The model under review builds one solid part; all positions refer to its coordinate system, in mm. Coordinates: 2 decimals unless noted, no trailing zeros. Order: outer loops, then holes, each group sorted by start corner. A loop starts at its lowest first (then second) coordinate and runs counter-clockwise, first axis right, second up. Notation, with made-up numbers: (-29, -3) - (30, -3) arc R20 ccw to (30, 1) - close; hole circle Ø11 at (49.5, 29). An arc over 180 degrees is marked (long way). Answer in a Markdown table with one row per item.
Autodesk Inventor part; units mm, degrees
ref_plane "YZ Plane" through (0, 0, 0) normal (1, 0, 0) x (0, 1, 0)
ref_plane "XZ Plane" through (0, 0, 0) normal (0, 1, 0) x (-1, 0, 0)
ref_plane "XY Plane" through (0, 0, 0) normal (0, 0, 1) x (1, 0, 0)
sketch "Náčrt1" plane through (3.6, 12.9231, 50.0016) normal (0, 0, 1) x (1, 0, 0)
  line L0 (3.4, -51.2206) -> (3.4, 32.0765)
  line L1 (-10.6, 32.0765) -> (-10.6, -51.2206)
  line L2 (3.4, 32.0765) -> (-10.6, 32.0765)
  circle A0 centre (-3.5987, -48.8454) radius 2.0783
  line L3 (0, -50.927) -> (0, 0)
  line L4 (-3.6, -53.0054) -> (0, -50.927)
  line L5 (-7.2, -50.927) -> (-3.6, -53.0054)
  arc A1 (-10.6, -50.9238) -> (3.4, -50.787) centre (-3.5993, -50.9238) ccw
  line L6 (3.4, -25.4635) -> (3.4, -18.4635)
  line L7 (3.4, -18.4635) -> (23.4, -18.4635)
  line L8 (23.4, -18.4635) -> (23.4, -32.4635)
  line L9 (23.4, -32.4635) -> (3.4, -32.4635)
  line L10 (3.4, -25.4635) -> (3.4, -32.4635)
  line L11 (23.4, -25.4635) -> (23.4, -22.9635)
  line L12 (23.4, -22.9635) -> (26.9, -22.9635)
  line L13 (26.9, -22.9635) -> (26.9, -27.9635)
  line L14 (26.9, -27.9635) -> (23.4, -27.9635)
  line L15 (23.4, -25.4635) -> (23.4, -27.9635)
  line L16 (35.5188, -25.4635) -> (33.2094, -29.4635)
  line L17 (33.2094, -29.4635) -> (28.5906, -29.4635)
  line L18 (28.5906, -29.4635) -> (27.7246, -27.9635)
  line L19 (27.7246, -22.9635) -> (28.5906, -21.4635)
  line L20 (28.5906, -21.4635) -> (33.2094, -21.4635)
  line L21 (33.2094, -21.4635) -> (35.5188, -25.4635)
  line L22 (26.9, -22.9635) -> (27.7246, -22.9635)
  line L23 (26.9, -27.9635) -> (27.7246, -27.9635)
  line L24 (-10.6, -25.4635) -> (-10.6, -18.4635)
  line L25 (-10.6, -18.4635) -> (-30.6, -18.4635)
  line L26 (-30.6, -18.4635) -> (-30.6, -32.4635)
  line L27 (-30.6, -32.4635) -> (-10.6, -32.4635)
  line L28 (-10.6, -25.4635) -> (-10.6, -32.4635)
  line L29 (-30.6, -25.4635) -> (-30.6, -22.9635)
  line L30 (-30.6, -25.4635) -> (-30.6, -27.9635)
  line L31 (-27.1, -27.9635) -> (-30.6, -27.9635)
  line L32 (-30.6, -22.9635) -> (-27.1, -22.9635)
  line L33 (-27.1, -22.9635) -> (-27.1, -27.9635)
  line L34 (-27.1, -22.9635) -> (-26.2754, -22.9635)
  line L35 (-27.1, -27.9635) -> (-26.2754, -27.9635)
  line L36 (-25.4094, -29.4635) -> (-26.2754, -27.9635)
  line L37 (-26.2754, -22.9635) -> (-25.4094, -21.4635)
  line L38 (-20.7906, -29.4635) -> (-25.4094, -29.4635)
  line L39 (-25.4094, -21.4635) -> (-20.7906, -21.4635)
  line L40 (-18.4812, -25.4635) -> (-20.7906, -29.4635)
  line L41 (-20.7906, -21.4635) -> (-18.4812, -25.4635)
  line L42 (-3.6, 32.0765) -> (-3.6, 46.0765)
  arc A2 (-31.8843, 17.7922) -> (24.6843, 17.7922) centre (-3.6, 46.0765) ccw
  line L43 (-3.6, 46.0765) -> (-31.8843, 17.7922)
  line L44 (-3.6, 46.0765) -> (24.6843, 17.7922)
  line L45 (-3.6, 46.0765) -> (48.0562, 46.0765) construction
  line L46 (-25.5203, 24.1562) -> (-23.7525, 25.9239)
  line L47 (-25.5203, 24.1562) -> (-27.2881, 22.3884)
  line L48 (-24.8132, 19.9135) -> (-27.2881, 22.3884)
  line L49 (-23.7525, 25.9239) -> (-21.2777, 23.4491)
  line L50 (-21.2777, 23.4491) -> (-24.8132, 19.9135)
  line L51 (-21.2777, 23.4491) -> (-20.6946, 22.866)
  line L52 (-24.8132, 19.9135) -> (-24.2301, 19.3305)
  line L53 (-20.6946, 22.866) -> (-19.0216, 23.3143)
  line L54 (-24.6784, 17.6574) -> (-24.2301, 19.3305)
  line L55 (-19.0216, 23.3143) -> (-15.7556, 20.0483)
  line L56 (-16.951, 15.5869) -> (-21.4124, 14.3914)
  line L57 (-15.7556, 20.0483) -> (-16.951, 15.5869)
  line L58 (-21.4124, 14.3914) -> (-24.6784, 17.6574)
  line L59 (26.8896, 32.7254) -> (28.085, 28.264)
  line L60 (22.4282, 33.9209) -> (26.8896, 32.7254)
  line L61 (28.085, 28.264) -> (24.819, 24.998)
  line L62 (19.1622, 30.6549) -> (22.4282, 33.9209)
  line L63 (18.3203, 24.1562) -> (16.5525, 25.9239)
  line L64 (19.6105, 28.9819) -> (19.1622, 30.6549)
  line L65 (24.819, 24.998) -> (23.146, 25.4463)
  line L66 (19.0274, 28.3988) -> (19.6105, 28.9819)
  line L67 (19.0274, 28.3988) -> (22.563, 24.8633)
  line L68 (22.563, 24.8633) -> (23.146, 25.4463)
  line L69 (22.563, 24.8633) -> (20.0881, 22.3884)
  line L70 (18.3203, 24.1562) -> (20.0881, 22.3884)
  line L71 (16.5525, 25.9239) -> (19.0274, 28.3988)
  line L72 (24.6843, 17.7922) -> (18.3203, 24.1562)
  circle A3 centre (-3.6, 46.0765) radius 5
  line L73 (-7.2, -50.927) -> (-7.2, 32.0765)
  line L74 (0, -50.927) -> (0, 32.0765)
  line L75 (-7.2, 29.2565) -> (-3.6, 32.0765)
  line L76 (-3.6, 32.0765) -> (0, 29.2565)
  line L77 (-3.6, 29.2565) -> (-1.5215, 29.2565) construction
  circle A4 centre (-3.6, 27.178) radius 2.0785
  line L78 (-5.6785, 27.1779) -> (-5.677, -48.8455)
  line L79 (-1.5215, 27.1779) -> (-1.5203, -48.8454)
  point P0 (30.9, -25.4635)
  point P1 (26.9, -25.4635)
  point P2 (-27.1, -25.4635)
  point P3 (-23.1, -25.4635)
  point P4 (-23.0454, 21.6813)
  point P5 (-20.217, 18.8529)
  point P6 (23.4958, 25.7125)
  point P7 (23.6236, 29.4595)
  point P8 (20.7952, 26.631)
  point P9 (-10.6, 6.6937)
  point P10 (3.4, 6.6937)
  point P11 (16.5525, 25.9239)
  point P12 (-0.0645, 42.5409)
  point P13 (-7.1355, 42.5409)
  dimension "d4" = 7
  dimension "d5" = 20
  dimension "k" = 14
  dimension "d9" = 3.5
  dimension "d10" = 5
  dimension "d14" = 8
  dimension "d15" = 4
  dimension "d16" = 7
  dimension "d19" = 14
  dimension "d21" = 45
  dimension "d22" = 40
  dimension "d24" = 10
  dimension "d34" = 4.1567
  dimension "d35" = 2.0817
  dimension "d36" = 2.82
extrude "Vysunutí1" add sketch "Náčrt1" against normal blind 4 contours A1 L1 A2 L73 L5 L4 L3 L74 L0 | A2 L74 L2 L0 | L74 L3 L4 L5 L73 A2 L78 A0 L79 | A2 L79 A4 L78 L73 L75 L76 L74 | L1 L2 L73 A2 | L74 L76 L2 | L79 A0 L78 A2 | A2 L78 A4 L79 | L75 L73 L2 | A4 | A0
extrude "Vysunutí2" cut sketch "Náčrt1" against normal blind 2.5 contours L74 L3 L4 L5 L73 A2 L78 A0 L79 | A2 L79 A4 L78 L73 L75 L76 L74 | L79 A0 L78 A2 | A2 L78 A4 L79 | A4 | A0
extrude "Vysunutí3" add sketch "Náčrt1" against normal blind 4 contours L0 L7 L8 L9 | L27 L26 L31 L35 L36 L38 L40 L41 L39 L37 L34 L32 L25 L1 | L8 L12 L13 L14 | L13 L22 L19 L20 L21 L16 L17 L18 L23
extrude "Vysunutí4" add sketch "Náčrt1" against normal blind 4 contours L0 L2 L42 A3 L44 A2 | A2 L43 L48 L52 L54 L58 L56 L57 L55 L53 L51 L49 A3 L42 L2 L1 | L44 L71 L67 L69 | L67 L66 L64 L62 L60 L59 L61 L65 L68
sketch "Náčrt2" plane through (3.6, 12.9231, 50.0016) normal (0, 0, 1) x (1, 0, 0)
  line L0 (-7.2, 0) -> (-3.6, 2.0785)
  line L1 (-3.6, 2.0785) -> (0, 0)
  arc A0 (-1.525, -2.1008) -> (-5.675, -2.1796) centre (-3.6012, -2.0791) ccw
  line L2 (-5.675, -2.1796) -> (-5.675, -48.7542)
  line L3 (-1.525, -48.7062) -> (-1.525, -2.1008)
  arc A1 (-5.675, -48.7542) -> (-1.525, -48.7062) centre (-3.5987, -48.8454) ccw
  line L4 (-3.6, -53.0054) -> (-7.2, -50.927)
  line L5 (-7.2, -50.927) -> (-7.2, 0)
  line L6 (0, -50.927) -> (-3.6, -53.0054)
  line L7 (0, 29.2565) -> (0, -50.927)
  line L8 (-7.2, 35) -> (-3.6, 37.0785)
  line L9 (-3.6, 37.0785) -> (0, 35)
  line L10 (-7.2, 0) -> (-7.2, 35)
  line L11 (0, 0) -> (0, 35)
  circle A2 centre (-3.6012, -2.0791) radius 2.0763
  circle A3 centre (-3.601, 32.9202) radius 2.0763
  line L12 (-3.6406, -0.0032) -> (-3.6, 2.0785)
  line L13 (-5.675, -2.1796) -> (-5.6773, 32.9201)
  line L14 (-1.525, -2.1008) -> (-1.5247, 32.9202)
  line L15 (-7.2, 0) -> (-5.6752, 0.8803)
  line L16 (-5.6752, 0.8803) -> (-3.6, 2.0785)
  line L17 (-3.6, 2.0785) -> (-1.525, 0.8804)
  line L18 (-1.525, 0.8804) -> (0, 0)
  point P0 (-3.6, -12.9231)
  dimension "d27" = 35
  dimension "d28" = 37.0817
  dimension "d" = 4.1525
  dimension "d30" = 4.1525
  dimension "d31" = 4.1583
  dimension "d32" = 3.6012
  dimension "d33" = 3.601
extrude "Vysunutí5" cut sketch "Náčrt1" against normal through all contours L79 A0 L78 A2 | A2 L78 A4 L79 | A4 | A0
equation "\"d30\" = d"
properties part number "New_08_Crane_Arm_Vertical_XL"
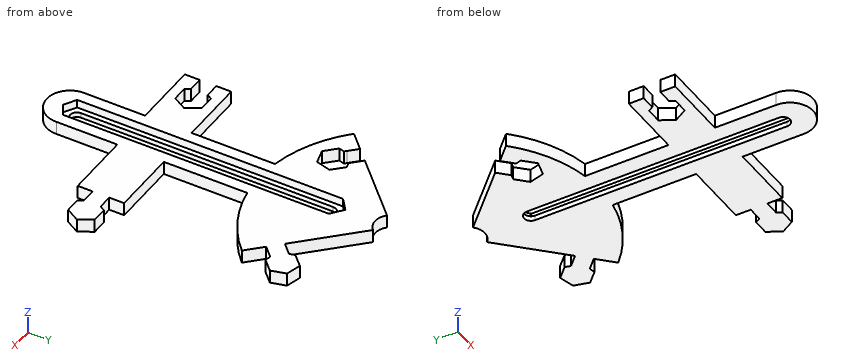
Item 1: To check wall thickness, follow line 1 (X direction, y = -23.5, z = 46.2); line 2 (X direction, y = 15, z = 48.6); line 3 (Y direction, x = -13.5, z = 46.6). State the ranges of each line that lie inside material, in increasing order. Write a range as from..to.
Check values:
| item | result |
|---|---|
| line 1 | -7..-2.08, 2.08..7 |
| line 2 | -7..-3.6, 3.6..7 |
| line 3 | -19.54..-5.54, 21.35..28.47, 34.32..45.5 |
Item 2: Clearance check with flat-ended pins moving along their axes: pin 1 Ø1 at (x, z) = (-9, 49.5) entering from +Y; pin 2 Ø1.2 at (x, z) = (35, 47) entering from -Y; pin 3 Ø2 at (x, z) = (-6, 46.5) entering from -Y. State where each tip first meets the part, or that it passes through.
Check values:
| item | result |
|---|---|
| pin 1 | y = 50.5 |
| pin 2 | y = -16.54 |
| pin 3 | y = -42.9 |
Item 3: We need section B-B, the plane x = -9. Write out the cut boundary in (y, z), then the cut area to 3 significant figures.
Check values:
| item | result |
|---|---|
| outline | (-19.54, 46) - (-5.54, 46) - (-5.54, 50) - (-19.54, 50) - close; (20.03, 46) - (50, 46) - (50, 50) - (20.03, 50) - close |
| area | 176 mm^2 |
Item 4: We need section C-C, the plane y = -39. Write out the cut boundary in (x, z), then the cut area to 3 significant figures.
Check values:
| item | result |
|---|---|
| outline | (-6.93, 46) - (6.93, 46) - (6.93, 50) - (1.87, 50) - (1.87, 47.5) - (-1.87, 47.5) - (-1.87, 50) - (-6.93, 50) - close |
| area | 46.1 mm^2 |
Item 5: We need section A-A, the plane y = 10. Write out the cut boundary in (x, z).
Check values:
| item | result |
|---|---|
| outline | (-7, 46) - (-2.08, 46) - (-2.08, 47.5) - (-3.6, 47.5) - (-3.6, 50) - (-7, 50) - close; (2.08, 46) - (7, 46) - (7, 50) - (3.6, 50) - (3.6, 47.5) - (2.08, 47.5) - close |
Item 6: We need section D-D, the plane x = 5. Write out the cut boundary in (y, z), then the cut area to 3 significant figures.
Check values:
| item | result |
|---|---|
| outline | (-42.9, 46) - (54, 46) - (54, 50) - (-42.9, 50) - close |
| area | 388 mm^2 |
